from build123d import *

# Parameters (mm, degrees)
F0_W     = 8.849032
F0_H     = 1.659194
F1_DEPTH = 6.604
F2_DEPTH = 2.54


with BuildPart() as f1:
    # F0 (on Front) → F1 (new body)
    with BuildSketch(Plane.XZ):
        with BuildLine():
            add(Edge.make_bspline(
                [(-66.073255, -37.148017), (-72.320135, -20.923742), (-73.008267, -9.742427), (-67.282905, 2.894996)],
                knots=[0, 0, 0, 0, 40.06128, 40.06128, 40.06128, 40.06128], degree=3))
            Line((-66.073255, -37.148017), (26.679299, -37.148017))
            Line((26.679299, -37.148017), (26.654679, -9.997438))
            ThreePointArc((26.654679, -9.997438), (26.497353, -8.016108), (26.032825, -6.083588))
            Line((26.032825, -6.083588), (20.713379, 10.284061))
            ThreePointArc((20.713379, 10.284061), (19.292549, 5.138633), (14.448968, 2.894996))
            Line((14.448968, 2.894996), (-67.282905, 2.894996))
        make_face()
        with Locations((12.289253, -8.810178)):
            Rectangle(F0_W, F0_H, mode=Mode.SUBTRACT)
    extrude(amount=-F1_DEPTH)

    # F0 (on Front) → F2 (join)
    with BuildSketch(Plane.XZ):
        with BuildLine():
            add(Edge.make_bspline(
                [(-66.073255, -37.148017), (-72.320135, -20.923742), (-73.008267, -9.742427), (-67.282905, 2.894996)],
                knots=[0, 0, 0, 0, 40.06128, 40.06128, 40.06128, 40.06128], degree=3))
            Line((-66.073255, -37.148017), (26.679299, -37.148017))
            Line((26.679299, -37.148017), (26.654679, -9.997438))
            ThreePointArc((26.654679, -9.997438), (26.497353, -8.016108), (26.032825, -6.083588))
            Line((26.032825, -6.083588), (20.713379, 10.284061))
            ThreePointArc((20.713379, 10.284061), (19.292549, 5.138633), (14.448968, 2.894996))
            Line((14.448968, 2.894996), (-67.282905, 2.894996))
        make_face()
        with Locations((12.289253, -8.810178)):
            Rectangle(F0_W, F0_H, mode=Mode.SUBTRACT)
        with BuildLine():
            Line((-47.033889, 25.107424), (-67.282905, 2.894996))
            Line((-67.282905, 2.894996), (14.448968, 2.894996))
            ThreePointArc((14.448968, 2.894996), (19.292549, 5.138633), (20.713379, 10.284061))
            Line((20.713379, 10.284061), (18.791883, 21.868555))
            ThreePointArc((18.791883, 21.868555), (16.633835, 25.673071), (12.527472, 27.17949))
            Line((12.527472, 27.17949), (-42.341152, 27.17949))
            ThreePointArc((-42.341152, 27.17949), (-44.906071, 26.638422), (-47.033889, 25.107424))
        make_face()
    extrude(amount=-F2_DEPTH)


solid = f1.part
Geometry check sheet. Reference: the model listing, model coordinates, mm. A direction names the side the tool comes from. Round coordinates to 2 decimals unless told otherwise and drop trailing zeros. Write each loop counter-clockwise with the first axis right and the second up, starting at its lowest first coordinate (ties: lowest second). Pieces come first, ordered by that corner, then holes.
Item 1: Section check B-B (z = 4.5). Record the boundary of the cut face in (x, y).
Determined:
outline: (-65.82, 0) - (22.59, 0) - (22.59, 6.6) - (18.67, 6.6) - (18.67, 2.54) - (-65.82, 2.54) - close
Item 2: Section check C-C (z = 12). Record the boundary of the cut face in (x, y), plus the area to 3 significant figures.
Determined:
outline: (-58.98, 0) - (20.43, 0) - (20.43, 2.54) - (-58.98, 2.54) - close
area: 202 mm2
Item 3: Access from +Z, -Z, +X, -X, +Y, -Y to the whole of each face (thin tool, end or side, straight path). Record for faces 1 (the face through (-20, 3, -37.148)), 2 (the face through (-26, 5, 2.895)), 3 (the face through (19.342, 4.544, 5.198)), 4 (the face through (12, 3, -7.981)).
Determined:
face 1: -Z, +X, -X, +Y, -Y
face 2: +Z, -X, +Y
face 3: -X, +Y
face 4: +Y, -Y
Item 4: Material ranges on line 1 along Z through (x, y) = (9, 3) (3 decimals); line 2 along Z through (x, y) = (13, 2.5); line 3 along Y through (x, z) = (-11, 6), recorded low to high.
Determined:
line 1: z = -37.148 to -9.64, -7.981 to 2.895
line 2: z = -37.15 to -9.64, -7.98 to 27.16
line 3: y = 0 to 2.54
Item 5: Go/stop test with flat-tipped pins: pin 1 Ø12 at (x, z) = (-50.5, 3.5) entering from -Y; pin 2 Ø1.3 at (y, z) = (2.5, -9) entering from -X; pin 3 Ø1.3 at (y, z) = (2, -9) entering from +X; pin 4 Ø1.5 at (x, y) = (-53, 2) entering from +Z. Record where each tip stops, or that it passes through.
Determined:
pin 1: stops at y = 0
pin 2: stops at x = -70.92
pin 3: stops at x = 26.65
pin 4: stops at z = 19.39
Item 6: Section check A-A (x = -63.5). Record the boundary of the cut face in (y, z) (3 decimals).
Determined:
outline: (0, -37.148) - (6.604, -37.148) - (6.604, 2.895) - (2.54, 2.895) - (2.54, 7.045) - (0, 7.045) - close
Item 7: Mould release check, pull along Z, two halves, no side actions. Record for faces 5 (the face through (12, 3, -9.64)), 6 (the face through (-22, 0, -5)), 7 (the face through (26.5, 3.26, -8.04)): +Z half, -Z half, draft (parallel to the pull), parting line (faces both ways), or undercut.
Determined:
face 5: undercut
face 6: draft
face 7: +Z half
